Source: CAD feature listing. Evaluate the final solid. Frame: model axes, mm. Give positions to 0.01 mm unless a question says otherwise; leave off trailing zeros. Order: outer loops, then holes, each group sorted by start corner. A loop starts at its lowest first (then second) coordinate and runs counter-clockwise, first axis right, second up. Notation, with made-up numbers: (25, 2) - (45, 2) arc R31 cw to (45, 35) - close; hole circle Ø4 at (-8, -36.5). An arc over 180 degrees is marked (long way). Use CSV: the item, a comma, the result in double quotes.
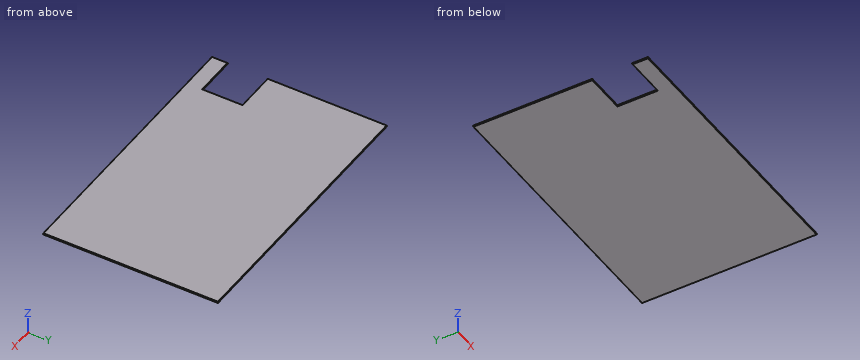
```python
from build123d import *

# Parameters (mm, degrees)
F0_W     = 906
F0_H     = 575
F1_DEPTH = 2.5
F2_W     = 1
F2_H     = 131
F2_W_2   = 135
F3_DEPTH = 5.001
F4_SIZE  = 1


with BuildPart() as f1:
    # F0 (on Top) → F1 (new body, symmetric)
    with BuildSketch(Plane.XY):
        Rectangle(F0_W, F0_H)
    extrude(amount=F1_DEPTH, both=True)

    # F2 (on face) → F3 (cut, through all)
    with BuildSketch(Plane.XY.offset(2.5)):
        with Locations((-453.5, -170)):
            Rectangle(F2_W, F2_H)
        with Locations((-385.5, -170)):
            Rectangle(F2_W_2, F2_H)
    extrude(amount=-F3_DEPTH, mode=Mode.SUBTRACT)

    # F4
    f4_edges = [f1.edges().sort_by_distance(p)[0] for p in [
        (-453, 91.5, 2.5),
        (-453, 91.5, -2.5),
        (-453, -261.5, -2.5),
        (-453, -261.5, 2.5),
        (0, -287.5, -2.5),
        (0, -287.5, 2.5),
        (453, 0, 2.5),
        (453, 0, -2.5),
        (0, 287.5, 2.5),
        (0, 287.5, -2.5),
        (-385.5, -104.5, 2.5),
        (-385.5, -104.5, -2.5),
        (-318, -170, -2.5),
        (-318, -170, 2.5),
        (-385.5, -235.5, 2.5),
        (-385.5, -235.5, -2.5),
    ]]
    chamfer(f4_edges, length=F4_SIZE)


solid = f1.part
```
Item 1: First-contact query: pin 1 (0.9 mm diameter, centred on y = -179.5, z = 0.5, fed in from -X). Flat tip, straight axial feed; report the tip coordinate or a pass-through.
Filled in:
pin 1,"stops at x = -318"
Item 2: Section A-A on z = 0.25. Return the cut outline in (x, y), then the cut area to 3 significant figures.
Filled in:
outline,"(-453, -287.5) - (453, -287.5) - (453, 287.5) - (-453, 287.5) - (-453, -104.5) - (-318, -104.5) - (-318, -235.5) - (-453, -235.5) - close"
area,"503,000 mm2"
Item 3: Section B-B on y = -202. Return the cut outline in (x, z).
Filled in:
outline,"(-318, -1.5) - (-317, -2.5) - (452, -2.5) - (453, -1.5) - (453, 1.5) - (452, 2.5) - (-317, 2.5) - (-318, 1.5) - close"
Item 4: Material intervals for line 1 (Y direction, x = -392, z = 1.1); line 2 (X direction, y = -152.5, z = -0.1); line 3 (Y direction, x = 192, z = 2.3), sorted ascending. Write a range as from..to.
Filled in:
line 1,"y = -287.5..-235.5, -104.5..287.5"
line 2,"x = -318..453"
line 3,"y = -286.7..286.7"
